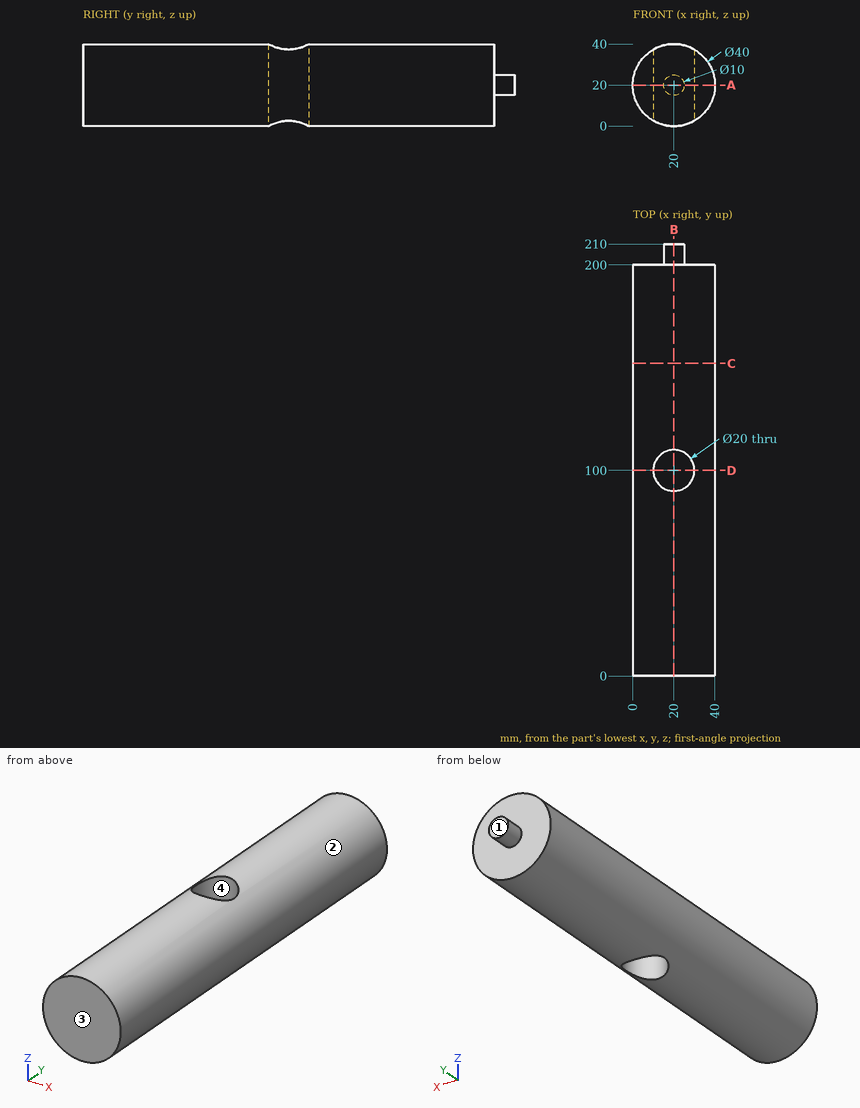
Can you work these out from the drawing? Everything is in mm from the part's minimum corner. Round coordinates to 2 decimals unless told otherwise and drop trailing zeros. Write each loop counter-clockwise with the first axis right and the second up, starting at its lowest first coordinate (ties: lowest second). Pieces come first, ordered by that corner, then holes. Notation, with made-up numbers: (42.5, 44.25) - (95.5, 44.25) arc R19 ccw to (95.5, 75.25) - close; hole circle Ø5 at (24, 42.5). An arc over 180 degrees is marked (long way). Put each result on its own line as item: value. Start each with the question number.
(1) Will these pins go through, and if not, where does the flat tip stop? pin 1 (4 mm diameter, centred on x = 29, y = 74.5, fed in from -Z) (3 decimals); pin 2 (5 mm diameter, centred on x = 27.5, z = 18.5, fed in from +Y); pin 3 (4 mm diameter, centred on y = 44.5, z = 21, fed in from -X).
(2) I want a section at B-B, the plane x = 20. Please give me the cut outline in (y, z).
(3) Thinking about a two-plate mould opening in Y: for the marked faces 1, 2, 3 and 4, which applies, released by +Y, released by -Y, zero draft, split by the parting line, or undercut?
(4) I want a section at D-D, the plane y = 100. Please give me the cut outline in (x, z), plus the area to 3 significant figures.
(5) I need wall thicknesses on probe 1 along Y at (x, z) = (6, 30); probe 2 along Y at (x, z) = (20.5, 4.5); probe 3 along X at (y, z) = (100, 15.5). Which ranges of each line are inside material? Lowest first, please.
(6) I want a section at A-A, the plane z = 20. Please give me the cut outline in (x, y), plus the area to 3 significant figures.
(7) I want a section at C-C, the plane y = 152. Please give me the cut outline in (x, z), plus the area to 3 significant figures.
Here are the results:
1. pin 1: stops at z = 1.265
1. pin 2: stops at y = 200
1. pin 3: stops at x = 0
2. outline: (0, 0) - (90, 0) - (90, 40) - (0, 40) - close; (110, 0) - (200, 0) - (200, 15) - (210, 15) - (210, 25) - (200, 25) - (200, 40) - (110, 40) - close
3. face 1: released by +Y
3. face 2: zero draft
3. face 3: released by -Y
3. face 4: undercut
4. outline: (10, 2.68) - (10, 37.32) arc R20 ccw to start; (30, 2.68) arc R20 ccw to (30, 37.32) - close
4. area: 491 mm^2
5. probe 1: y = 0 to 200
5. probe 2: y = 0 to 90.01, 109.99 to 200
5. probe 3: x = 0.51 to 10, 30 to 39.49
6. outline: (0, 0) - (40, 0) - (40, 200) - (25, 200) - (25, 210) - (15, 210) - (15, 200) - (0, 200) - close; hole circle Ø20 at (20, 100)
6. area: 7,790 mm^2
7. outline: circle Ø40 at (20, 20)
7. area: 1,260 mm^2
